Design review of the part built by this model. Coordinates are the model's own, in mm. Coordinates: 2 decimals unless noted, no trailing zeros. Write each loop counter-clockwise with the first axis right and the second up, starting at its lowest first coordinate (ties: lowest second). Pieces come first, ordered by that corner, then holes.
Q1. Take a section at A-A (y = 1.95). Give the boundary of the cut face in (x, z).
Q2. Insertion check: pin 1 (1.5 mm diameter, centred on y = 1, z = -13, fed in from -X); pin 2 (0.8 mm diameter, centred on y = 1, z = -58, fed in from +X); pin 3 (0.8 mm diameter, centred on x = 75, y = 0.5, fed in from +Z); pin 4 (4 mm diameter, centred on x = 10, z = -12, fed in from -Y). Each pin has a flat end and moves straight along its axis. Give the tip position at first contact, or say it passes through.
Q3. For probe 1 along X at (y, z) = (0.4, -48), list the stretches that pass through material, from the lowest coordinate up.
Q4. Take a section at B-B (z = -7). Give the boundary of the cut face in (x, y).
```python
from build123d import *

# Parameters (mm, degrees)
SKETCH1_W           = 76.2
SKETCH1_H           = 63.5
BOSS_EXTRUDE1_DEPTH = 2.54
SKETCH2_W           = 2.54
SKETCH2_H           = 19.8966582
CUT_EXTRUDE1_DEPTH  = 3.54
SKETCH3_W           = 2.54
SKETCH3_H           = 22.4366582
SKETCH3_H_2         = 19.8966582
CUT_EXTRUDE2_DEPTH  = 3.54


with BuildPart() as part:
    # Sketch1 → Boss-Extrude1 (new body)
    with BuildSketch(Plane(origin=(0, 0, 0), x_dir=(1, 0, 0), z_dir=(0, 1, 0))):
        with Locations((38.1, 31.75)):
            Rectangle(SKETCH1_W, SKETCH1_H)
    extrude(amount=BOSS_EXTRUDE1_DEPTH)

    # Sketch2 → Cut-Extrude1 (cut, through all)
    with BuildSketch(Plane(origin=(0, 2.54, 0), x_dir=(1, 0, 0), z_dir=(0, 1, 0))):
        with Locations((1.27, 53.5516709)):
            Rectangle(SKETCH2_W, SKETCH2_H)
    extrude(amount=-CUT_EXTRUDE1_DEPTH, mode=Mode.SUBTRACT)

    # Sketch3 → Cut-Extrude2 (cut, through all)
    with BuildSketch(Plane(origin=(0, 2.54, 0), x_dir=(1, 0, 0), z_dir=(0, 1, 0))):
        with Locations((1.27, 11.2183291)):
            Rectangle(SKETCH3_W, SKETCH3_H)
        with Locations((74.93, 53.5516709)):
            Rectangle(SKETCH3_W, SKETCH3_H_2)
        with Locations((74.93, 11.2183291)):
            Rectangle(SKETCH3_W, SKETCH3_H)
    extrude(amount=-CUT_EXTRUDE2_DEPTH, mode=Mode.SUBTRACT)


solid = part.part
```
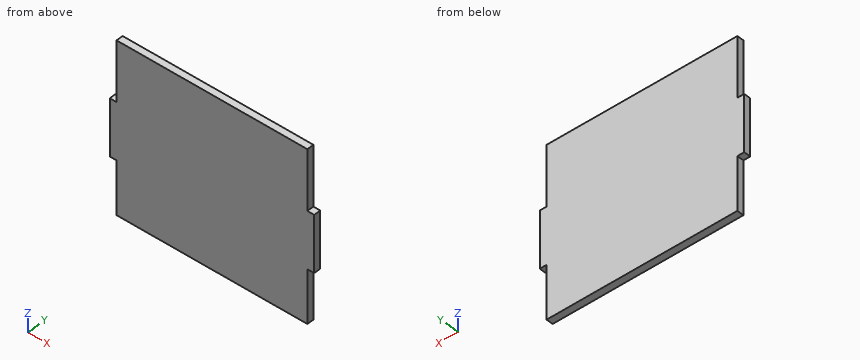
Response:
1. outline: (0, -43.6) - (2.54, -43.6) - (2.54, -63.5) - (73.66, -63.5) - (73.66, -43.6) - (76.2, -43.6) - (76.2, -22.44) - (73.66, -22.44) - (73.66, 0) - (2.54, 0) - (2.54, -22.44) - (0, -22.44) - close
2. pin 1: stops at x = 2.54
2. pin 2: stops at x = 73.66
2. pin 3: stops at z = -22.44
2. pin 4: stops at y = 0
3. probe 1: x = 2.54 to 73.66
4. outline: (2.54, 0) - (73.66, 0) - (73.66, 2.54) - (2.54, 2.54) - close
